The model under review builds one solid part; all positions refer to its coordinate system, in mm. A direction names the side the tool comes from. Coordinates: 2 decimals unless noted, no trailing zeros. Loops run counter-clockwise (first coordinate to the right, second up) from the corner with the lowest first, then second, coordinate; pieces in that order, holes last. Notation, with made-up numbers: (34, -3) - (54, -3) arc R5 cw to (54, 6) - close; hole circle Ø6 at (72.5, 27). An arc over 180 degrees is marked (long way). Use a Markdown table: item, result. Add a question column.
1) The part is to be moulded in two halves that separate along X. For faces 1 (the cylindrical face through (-280.094, 23.051, 330.811)), 2 (the flat face through (-288, -29, 335.426)), 3 (the flat face through (-320.3, 23.83, 290.86)), say which applies: pulls with the +X half, pulls with the -X half, needs draft (parallel to the pull), parting line crosses it, or undercut.
2) Add section C-C, the plane x = -330. Give the boundary of the cut face in (y, z), and give its area (3 significant figures).
3) To check wall thickness, follow L1, parallel to Y at x = -299.5, z = 299; L2, parallel to X at y = 4, z = 306; L3, parallel to Y at x = -273.5, z = 269. State the ranges of each line that lie inside material, in increasing order. Write a range as [from, to].
4) Add section B-B, the plane y = 8. Give the boundary of the cut face in (x, z), and give its area (4 significant figures).
5) Clearance check with flat-ended pins moving along their axes: pin 1 (2 mm diameter, centred on y = -27.5, z = 266, fed in from +X); pin 2 (4 mm diameter, centred on y = -20, z = 291, fed in from -X); pin 3 (3 mm diameter, centred on y = -22, z = 273.5, fed in from -X). State where each tip first meets the part, or that it passes through.
6) Add section A-A, the plane y = -31. Give the boundary of the cut face in (x, z), and give its area (3 significant figures).
7) For faces 4 (the flat face through (-259, -33.899, 300)), 5 (the cylindrical face through (-285.84, -23.96, 262.98)), 6 (the flat face through (-273, -19.899, 270)), list the 3-axis set-ups (+Z, -Z, +X, -X, +Y, -Y) from which the entire face can be reached by the end or side of a thin tool; tool diameter is ignored.
```python
from build123d import *

# Parameters (mm, degrees)
SKETCH2_W                                         = 62.3
SKETCH2_H                                         = 73.3
BOSS_EXTRUDE1_DEPTH                               = 3
BOSS_EXTRUDE3_DEPTH                               = 10
BOSS_EXTRUDE4_DEPTH                               = 48.2
SKETCH13_W                                        = 52.3
SKETCH13_H                                        = 47.3
BOSS_EXTRUDE5_DEPTH                               = 5
CUT_EXTRUDE2_REACH                                = 475.855
CSK_FOR_M3_FLAT_HEAD_MACHINE_SCREW1_D             = 3.4
CSK_FOR_M3_FLAT_HEAD_MACHINE_SCREW1_DEPTH         = 5
CSK_FOR_M3_FLAT_HEAD_MACHINE_SCREW1_CSINK_D       = 6.3
CSK_FOR_M3_FLAT_HEAD_MACHINE_SCREW1_CSINK_ANGLE   = 90
CHAMFER1_SIZE                                     = 1
BOSS_EXTRUDE7_DEPTH                               = 20
BOSS_EXTRUDE6_START                               = -6
BOSS_EXTRUDE6_OUTLINE_W                           = 14
BOSS_EXTRUDE6_OUTLINE_H                           = 20.4
BOSS_EXTRUDE6_DEPTH                               = 6
CHAMFER5_SIZE                                     = 10
CHAMFER2_SIZE                                     = 4
CSK_FOR_6_FLAT_HEAD_MACHINE_SCREW_100_D           = 3.7973
CSK_FOR_6_FLAT_HEAD_MACHINE_SCREW_100_CSINK_D     = 7.0866
CSK_FOR_6_FLAT_HEAD_MACHINE_SCREW_100_CSINK_ANGLE = 100
CHAMFER3_SIZE                                     = 1
F_3_0MM_DOWEL_HOLE1_D                             = 3.5
F_3_32_0_140625_DOWEL_HOLE1_D                     = 3.571875
HOLE4_D                                           = 5.64
HOLE4_DEPTH                                       = 4.2
CUT_EXTRUDE3_DEPTH                                = 4.2
CHAMFER4_SIZE                                     = 0.2


# Read off the part's stored shape, not the designer's step: Boss-Extrude6
with BuildPart() as part:
    # Sketch2 → Boss-Extrude1 (new body)
    with BuildSketch(Plane(origin=(0, -39.89907595, 0), x_dir=(1, 0, 0), z_dir=(0, 1, 0))):
        with Locations((-296.943004764, -298.776222799)):
            Rectangle(SKETCH2_W, SKETCH2_H)
    extrude(amount=BOSS_EXTRUDE1_DEPTH)

    # Sketch4 → Boss-Extrude3 (add)
    with BuildSketch(Plane(origin=(0, -36.89907595, 0), x_dir=(1, 0, 0), z_dir=(0, 1, 0))):
        Polygon((-323.093004764, -262.126222799), (-303.943004764, -262.126222799), (-303.943004764, -282.526222799), (-289.943004764, -282.526222799), (-289.943004764, -262.126222799), (-270.793004764, -262.126222799), (-270.793004764, -335.426222799), (-323.093004764, -335.426222799), align=None)
    extrude(amount=BOSS_EXTRUDE3_DEPTH)

    # Sketch5 → Boss-Extrude4 (add)
    with BuildSketch(Plane(origin=(0, -26.89907595, 0), x_dir=(1, 0, 0), z_dir=(0, 1, 0))):
        Polygon((-270.793004764, -288.126222799), (-323.093004764, -288.126222799), (-323.093004764, -335.426222799), (-318.093004764, -335.426222799), (-318.093004764, -293.126222799), (-275.793004764, -293.126222799), (-275.793004764, -335.426222799), (-270.793004764, -335.426222799), align=None)
    extrude(amount=BOSS_EXTRUDE4_DEPTH)

    # Sketch13 → Boss-Extrude5 (add)
    with BuildSketch(Plane(origin=(0, 21.30092405, 0), x_dir=(1, 0, 0), z_dir=(0, 1, 0))):
        with Locations((-296.943004764, -311.776222799)):
            Rectangle(SKETCH13_W, SKETCH13_H)
    extrude(amount=BOSS_EXTRUDE5_DEPTH)

    # Sketch15 → Cut-Extrude2 (cut, up to next)
    with BuildSketch(Plane(origin=(0, 26.30092405, 0), x_dir=(1, 0, 0), z_dir=(0, 1, 0)), mode=Mode.PRIVATE) as cut_extrude2_sk1:
        with BuildLine():
            Line((-308.443004764, -314.276222799), (-308.443004764, -335.426222799))
            Line((-308.443004764, -335.426222799), (-285.443004764, -335.426222799))
            Line((-285.443004764, -335.426222799), (-285.443004764, -314.276222799))
            ThreePointArc((-285.443004764, -314.276222799), (-296.943004764, -302.776222799), (-308.443004764, -314.276222799))
        make_face()
    cut_extrude2_tool1 = extrude(cut_extrude2_sk1.sketch, amount=-CUT_EXTRUDE2_REACH, mode=Mode.PRIVATE) & part.part
    add(cut_extrude2_tool1.solids().sort_by_distance((-296.943005, 26.300924, 320.226042))[0], mode=Mode.SUBTRACT)

    # CSK for M3 Flat Head Machine Screw1
    with Locations(Plane(origin=(0, 26.30092405, 0), x_dir=(1, 0, 0), z_dir=(0, 1, 0))):
        with Locations((-312.443004764, -298.776222799), (-281.443004764, -298.776222799), (-281.443004764, -329.776222799), (-312.443004764, -329.776222799)):
            CounterSinkHole(CSK_FOR_M3_FLAT_HEAD_MACHINE_SCREW1_D / 2, CSK_FOR_M3_FLAT_HEAD_MACHINE_SCREW1_CSINK_D / 2, depth=CSK_FOR_M3_FLAT_HEAD_MACHINE_SCREW1_DEPTH, counter_sink_angle=CSK_FOR_M3_FLAT_HEAD_MACHINE_SCREW1_CSINK_ANGLE)

    # Chamfer1
    chamfer1_edges = [part.edges().sort_by_distance(p)[0] for p in [
        (-296.943004764, -26.89907595, 335.426222799),
        (-275.793004764, -2.79907595, 335.426222799),
        (-318.093004764, -2.79907595, 335.426222799),
        (-313.268004764, 21.30092405, 335.426222799),
        (-280.618004764, 21.30092405, 335.426222799),
        (-308.443004764, 21.30092405, 324.851222799),
        (-285.443004764, 21.30092405, 324.851222799),
        (-296.943004764, 21.30092405, 302.776222799),
    ]]
    chamfer(chamfer1_edges, length=CHAMFER1_SIZE)

    # Sketch28 → Boss-Extrude7 (add)
    with BuildSketch(Plane(origin=(-288.526747439, -39.89907595, 232.373479331), x_dir=(1, 0, 0), z_dir=(0, 1, 0))):
        with BuildLine():
            Line((29.783182259, -35.452743468), (29.783182259, -32.752743468))
            ThreePointArc((29.783182259, -32.752743468), (28.904502603, -30.631423124), (26.783182259, -29.752743468))
            Line((26.783182259, -29.752743468), (24.083182259, -29.752743468))
            Line((24.083182259, -29.752743468), (4.783182369, -29.752743468))
            ThreePointArc((4.783182369, -29.752743468), (2.661862025, -30.631423124), (1.783182369, -32.752743468))
            Line((1.783182369, -32.752743468), (1.783182259, -40.052743468))
            Line((1.783182259, -40.052743468), (1.783182259, -42.752743468))
            ThreePointArc((1.783182259, -42.752743468), (2.661861916, -44.874063811), (4.783182259, -45.752743468))
            Line((4.783182259, -45.752743468), (7.483182259, -45.752743468))
            Line((7.483182259, -45.752743468), (26.783182369, -45.752743468))
            ThreePointArc((26.783182369, -45.752743468), (28.904502712, -44.874063811), (29.783182369, -42.752743468))
            Line((29.783182369, -42.752743468), (29.783182259, -35.452743468))
        make_face()
    extrude(amount=BOSS_EXTRUDE7_DEPTH)

    # Boss-Extrude6 outline → Boss-Extrude6 (add)
    with BuildSketch(Plane.XZ.offset(39.89907595).offset(BOSS_EXTRUDE6_START)):
        with Locations((-296.943004764, 272.326222799)):
            Rectangle(BOSS_EXTRUDE6_OUTLINE_W, BOSS_EXTRUDE6_OUTLINE_H)
        with BuildLine():
            ThreePointArc((-258.743565179, 265.126222799), (-258.971926582, 263.978172502), (-259.622244836, 263.004902456))
            Line((-259.622244836, 263.004902456), (-245.793004764, 273.776222799))
            Line((-245.793004764, 273.776222799), (-245.793004764, 323.776222799))
            Line((-245.793004764, 323.776222799), (-265.793004764, 335.426222799))
            Line((-265.793004764, 335.426222799), (-270.793004764, 335.426222799))
            Line((-270.793004764, 335.426222799), (-270.793004764, 278.126222799))
            Line((-270.793004764, 278.126222799), (-261.74356507, 278.126222799))
            ThreePointArc((-261.74356507, 278.126222799), (-259.622244726, 277.247543143), (-258.74356507, 275.126222799))
            Line((-258.74356507, 275.126222799), (-258.743565179, 265.126222799))
        make_face()
        Polygon((-328.093004764, 262.126222799), (-323.093004764, 262.126222799), (-323.093004764, 335.426222799), (-328.093004764, 335.426222799), (-348.093004764, 323.776222799), (-348.093004764, 273.776222799), align=None)
    extrude(amount=BOSS_EXTRUDE6_DEPTH)

    # Chamfer5
    chamfer5_edges = [part.edges().sort_by_distance(p)[0] for p in [
        (-323.093004764, -30.39907595, 262.126222799),
    ]]
    chamfer(chamfer5_edges, length=CHAMFER5_SIZE)

    # Chamfer2
    chamfer2_edges = [part.edges().sort_by_distance(p)[0] for p in [
        (-270.793004764, -0.29907595, 288.126222799),
        (-323.093004764, -0.29907595, 288.126222799),
        (-296.943004764, 26.30092405, 288.126222799),
        (-323.093004764, 26.30092405, 311.776222799),
        (-270.793004764, 26.30092405, 311.776222799),
    ]]
    chamfer(chamfer2_edges, length=CHAMFER2_SIZE)

    # CSK for #6 Flat Head Machine Screw (100)1 (through all)
    with Locations(Plane(origin=(0, -33.89907595, 0), x_dir=(1, 0, 0), z_dir=(0, 1, 0))):
        with Locations((-338.093004764, -278.776222799), (-338.093004764, -318.776222799), (-255.793004764, -318.776222799), (-255.793004764, -278.776222799)):
            CounterSinkHole(CSK_FOR_6_FLAT_HEAD_MACHINE_SCREW_100_D / 2, CSK_FOR_6_FLAT_HEAD_MACHINE_SCREW_100_CSINK_D / 2, counter_sink_angle=CSK_FOR_6_FLAT_HEAD_MACHINE_SCREW_100_CSINK_ANGLE)

    # Chamfer3
    chamfer3_edges = [part.edges().sort_by_distance(p)[0] for p in [
        (-286.843284917, -26.89907595, 262.126222799),
        (-268.293004764, -33.89907595, 335.426222799),
        (-303.943004764, -26.89907595, 272.326222799),
        (-255.793004764, -33.89907595, 329.601222799),
        (-245.793004764, -33.89907595, 298.776222799),
        (-252.7076248, -33.89907595, 268.390562628),
        (-308.518004764, -26.89907595, 262.126222799),
        (-348.093004764, -33.89907595, 298.776222799),
        (-338.093004764, -33.89907595, 329.601222799),
        (-325.593004764, -33.89907595, 335.426222799),
        (-318.093004764, -33.89907595, 262.126222799),
        (-338.093004764, -33.89907595, 267.951222799),
        (-289.943004764, -26.89907595, 272.326222799),
        (-296.943004764, -26.89907595, 282.526222799),
        (-323.093004764, -26.89907595, 282.126222799),
        (-318.093004764, -26.89907595, 267.126222799),
    ]]
    chamfer(chamfer3_edges, length=CHAMFER3_SIZE)

    # Ø3.0mm Dowel Hole1 (through all)
    with Locations(Plane(origin=(0, -33.89907595, 0), x_dir=(1, 0, 0), z_dir=(0, 1, 0))):
        with Locations((-296.943004764, -272.326222799)):
            Hole(F_3_0MM_DOWEL_HOLE1_D / 2)

    # 3/32 (0.140625) Dowel Hole1 (through all)
    with Locations(Plane(origin=(0, -19.89907595, 0), x_dir=(1, 0, 0), z_dir=(0, 1, 0))):
        with Locations((-283.743565179, -275.126222799), (-261.743565179, -265.126222799)):
            Hole(F_3_32_0_140625_DOWEL_HOLE1_D / 2)

    # Hole4
    with Locations(Plane(origin=(0, -39.89907595, 0), x_dir=(-1, 0, 0), z_dir=(0, -1, 0))):
        with Locations((296.943004764, -272.326222799)):
            Hole(HOLE4_D / 2, depth=HOLE4_DEPTH)

    # Sketch36 → Cut-Extrude3 (cut)
    with BuildSketch(Plane.XZ.offset(39.89907595)):
        Polygon((-298.571132523, 275.146222799), (-295.314877005, 275.146222799), (-293.686749245, 272.326222799), (-295.314877005, 269.506222799), (-298.571132523, 269.506222799), (-300.199260282, 272.326222799), align=None)
    extrude(amount=-CUT_EXTRUDE3_DEPTH, mode=Mode.SUBTRACT)

    # Chamfer4
    chamfer4_edges = [part.edges().sort_by_distance(p)[0] for p in [
        (-296.943004764, -39.89907595, 275.146222799),
        (-299.385196402, -39.89907595, 273.736222799),
        (-299.385196402, -39.89907595, 270.916222799),
        (-296.943004764, -39.89907595, 269.506222799),
        (-294.500813125, -39.89907595, 270.916222799),
        (-294.500813125, -39.89907595, 273.736222799),
    ]]
    chamfer(chamfer4_edges, length=CHAMFER4_SIZE)


solid = part.part
```
From the geometry:
| question | item | result |
|---|---|---|
| 1 | face 1 | undercut |
| 1 | face 2 | needs draft |
| 1 | face 3 | pulls with the -X half |
| 2 | outline | (-39.9, 263.24) - (-34.9, 263.24) - (-33.9, 264.39) - (-33.9, 333.16) - (-34.9, 334.32) - (-39.9, 334.32) - close |
| 2 | area | 425 mm^2 |
| 3 | L1 | y = [-39.9, -26.9], [21.3, 26.3] |
| 3 | L2 | x = [-323.09, -318.09], [-275.79, -270.79] |
| 3 | L3 | y = [-39.9, -19.9] |
| 4 | outline | (-323.09, 292.13) - (-319.09, 288.13) - (-274.79, 288.13) - (-270.79, 292.13) - (-270.79, 335.43) - (-274.79, 335.43) - (-275.79, 334.43) - (-275.79, 293.13) - (-318.09, 293.13) - (-318.09, 334.43) - (-319.09, 335.43) - (-323.09, 335.43) - close |
| 4 | area | 667.5 mm^2 |
| 5 | pin 1 | stops at x = -258.74 |
| 5 | pin 2 | stops at x = -323.09 |
| 5 | pin 3 | stops at x = -286.74 |
| 6 | outline | (-323.09, 272.13) - (-313.09, 262.13) - (-303.94, 262.13) - (-303.94, 282.53) - (-289.94, 282.53) - (-289.94, 262.13) - (-261.74, 262.13) arc R3 ccw to (-258.74, 265.13) - (-258.74, 275.13) arc R3 ccw to (-261.74, 278.13) - (-270.79, 278.13) - (-270.79, 335.43) - (-323.09, 335.43) - close; hole circle Ø3.57 at (-283.74, 275.13); hole circle Ø3.57 at (-261.74, 265.13) |
| 6 | area | 3,670 mm^2 |
| 7 | face 4 | +Z, +X, +Y |
| 7 | face 5 | -Z, -X, +Y |
| 7 | face 6 | -Z, +X, -X, +Y |
